The model under review builds one solid part; all positions refer to its coordinate system, in mm. Face numbers are marked on the shaded views. A direction names the side the tool comes from. Round coordinates to 2 decimals unless told otherwise and drop trailing zeros. Loops run counter-clockwise (first coordinate to the right, second up) from the corner with the lowest first, then second, coordinate; pieces in that order, holes last. Notation, with made-up numbers: (46, 56) -> (94, 56) arc R16 cw to (94, 86) -> close; hole circle Ø11 at (69, 17.5). An arc over 180 degrees is marked (long way). Write each question's results on one line, items separated by ' | '. Start each with the question number.
Item 1: We need section C-C (y = 16.5). Give the boundary of the cut face in (x, z), and give its area (3 significant figures).
Item 2: We need section A-A (x = 63.5). Give the boundary of the cut face in (y, z), and give its area (3 significant figures).
Item 3: For L1, parallel to Y at x = 63.5, z = 3.2; L2, parallel to Z at x = 77, y = 24; L3, parallel to X at y = 6, z = 19, list the stretches that pass through material, from the lowest coordinate up. Write a range as from..to.
Item 4: Clearance check with flat-ended pins moving along their axes: pin 1 Ø5 at (x, y) = (70.5, 17.5) entering from +Z; pin 2 Ø2 at (x, z) = (97.5, 25.5) entering from +Y; pin 3 Ø1 at (x, z) = (65, 20.5) entering from +Y. State where each tip first meets the part, or that it passes through.
Item 5: Tool access review of the marked faces 1 and 2: name each direction out of +Z, -Z, +X, -X, +Y, -Y from which nothing blocks a thin tool from reaching the whole face with its end or side.
Item 6: We need section B-B (x = 85.5). Give the boundary of the cut face in (y, z).
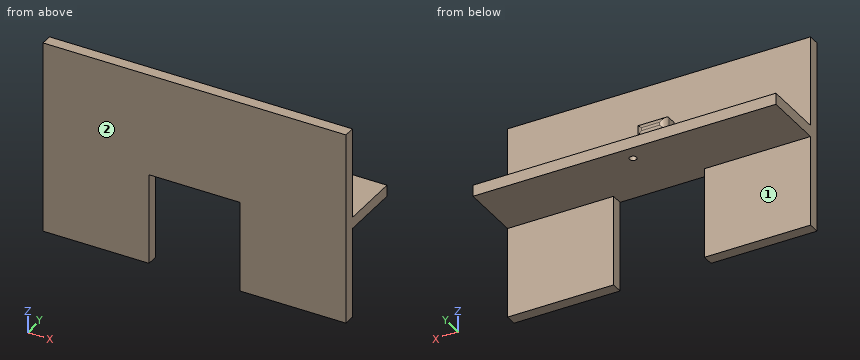
from build123d import *

# Parameters (mm, degrees)
SKETCH1_W           = 38.1
SKETCH1_H           = 4.7625
BOSS_EXTRUDE1_DEPTH = 127
SKETCH2_W           = 12.7
SKETCH2_H           = 6.35
BOSS_EXTRUDE2_DEPTH = 6.35
SKETCH3_R           = 1.499997
CUT_EXTRUDE1_DEPTH  = 138.389847924
FILLET1_R           = 2.54
SKETCH4_W           = 38.1
SKETCH4_H           = 38.1
CUT_EXTRUDE2_DEPTH  = 137.423436059


with BuildPart() as part:
    # Sketch1 → Boss-Extrude1 (new body)
    with BuildSketch(Plane(origin=(0, 0, 0), x_dir=(0, 0, -1), z_dir=(1, 0, 0))):
        Polygon((0, 30.1625), (0, 0), (-42.8625, 0), (-42.8625, 4.7625), (-4.7625, 4.7625), (-4.7625, 30.1625), align=None)
        with Locations((19.05, 2.38125)):
            Rectangle(SKETCH1_W, SKETCH1_H)
    extrude(amount=BOSS_EXTRUDE1_DEPTH)

    # Sketch2 → Boss-Extrude2 (add)
    with BuildSketch(Plane(origin=(0, 4.7625, 0), x_dir=(1, 0, 0), z_dir=(0, 1, 0))):
        with Locations((63.5, -20.6375)):
            Rectangle(SKETCH2_W, SKETCH2_H)
    extrude(amount=BOSS_EXTRUDE2_DEPTH)

    # Sketch3 → Cut-Extrude1 (cut, through all)
    with BuildSketch(Plane.XY.offset(4.7625)):
        with Locations((63.5, 23.8125)):
            Circle(SKETCH3_R)
    extrude(amount=-CUT_EXTRUDE1_DEPTH, mode=Mode.SUBTRACT)

    # Fillet1
    fillet1_edges = [part.edges().sort_by_distance(p)[0] for p in [
        (57.15, 11.1125, 20.6375),
        (63.5, 11.1125, 23.8125),
        (69.85, 11.1125, 20.6375),
        (63.5, 11.1125, 17.4625),
    ]]
    fillet(fillet1_edges, radius=FILLET1_R)

    # Sketch4 → Cut-Extrude2 (cut, through all)
    with BuildSketch(Plane(origin=(0, 4.7625, 0), x_dir=(1, 0, 0), z_dir=(0, 1, 0))):
        with Locations((63.5, 19.05)):
            Rectangle(SKETCH4_W, SKETCH4_H)
    extrude(amount=-CUT_EXTRUDE2_DEPTH, mode=Mode.SUBTRACT)


solid = part.part
Here are the results:
1) outline: (0, 0) -> (127, 0) -> (127, 4.76) -> (0, 4.76) -> close | area: 605 mm2
2) outline: (0, 0) -> (22.31, 0) -> (22.31, 4.76) -> (4.76, 4.76) -> (4.76, 17.46) -> (8.57, 17.46) arc R2.54 ccw to (11.11, 20) -> (11.11, 21.27) arc R2.54 ccw to (8.57, 23.81) -> (4.76, 23.81) -> (4.76, 42.86) -> (0, 42.86) -> close; (25.31, 0) -> (30.16, 0) -> (30.16, 4.76) -> (25.31, 4.76) -> close | area: 348 mm2
3) L1: y = 0..22.31, 25.31..30.16 | L2: z = 0..4.76 | L3: x = 57.15..69.85
4) pin 1: stops at z = 4.76 | pin 2: stops at y = 4.76 | pin 3: stops at y = 11.11
5) face 1: -Z, +X, -X, +Y | face 2: +Z, -Z, +X, -X, -Y
6) outline: (0, -38.1) -> (4.76, -38.1) -> (4.76, 0) -> (30.16, 0) -> (30.16, 4.76) -> (4.76, 4.76) -> (4.76, 42.86) -> (0, 42.86) -> close
